from build123d import *

# Parameters (mm, degrees)
F1_DEPTH = 0.5


with BuildPart() as f1:
    # F0 (on Top) → F1 (new body)
    with BuildSketch(Plane.XY):
        with BuildLine():
            ThreePointArc((4.5, 0), (0, -4.5), (-4.5, 0))
            Line((-4.5, 0), (-4.5, 4.834927))
            Line((-4.5, 4.834927), (-11.980261, 4.834927))
            Line((-11.980261, 4.834927), (-14.539381, 0))
            Line((-14.539381, 0), (-14.539381, -15))
            Line((-14.539381, -15), (0, -15))
            Line((0, -15), (14.539381, -15))
            Line((14.539381, -15), (14.539381, 0))
            Line((14.539381, 0), (11.980261, 4.834927))
            Line((11.980261, 4.834927), (4.5, 4.834927))
            Line((4.5, 4.834927), (4.5, 0))
        make_face()
    extrude(amount=F1_DEPTH)


solid = f1.part
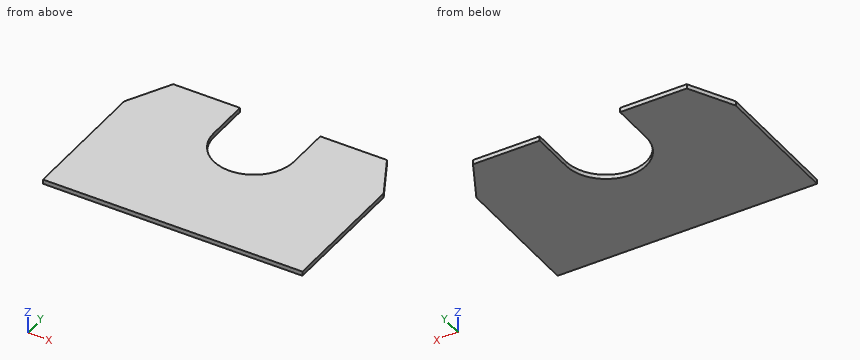
Model file for the job. Use its own axes, mm. Give positions to 0.01 mm unless a question says otherwise; leave off trailing zeros. Order: outer loops, then holes, each group sorted by start corner. A loop starts at its lowest first (then second) coordinate and runs counter-clockwise, first axis right, second up. Notation, with made-up numbers: (-17, 63) - (5, 63) arc R20 cw to (5, 67) - close; hole circle Ø5 at (51, 70.25). An arc over 180 degrees is marked (long way). Write item = value, one per line. Start each with the question number.
1. Cut at D-D, the plane y = -2.5. List the corners of the cut face in (x, z).
2. Probe line 1 along X through (y, z) = (2, 0.25); line 2 along X through (y, z) = (-4, 0.4); line 3 along Y through (x, z) = (-2, 0.15). List the from-to ranges inside material, lowest first.
3. Cut at C-C, the plane x = 0. List the corners of the cut face in (y, z).
4. Cut at A-A, the plane z = 0.35. List the corners of the cut face in (x, y), and give its area (3 significant figures).
5. Cut at B-B, the plane y = 1.25. List the corners of the cut face in (x, z), and give its area (3 significant figures).
Taken from the geometry:
q1.outline = (-14.54, 0) - (-3.74, 0) - (-3.74, 0.5) - (-14.54, 0.5) - close; (3.74, 0) - (14.54, 0) - (14.54, 0.5) - (3.74, 0.5) - close
q2.line_1 = -13.48 to -4.5, 4.5 to 13.48
q2.line_2 = -14.54 to -2.06, 2.06 to 14.54
q2.line_3 = -15 to -4.03
q3.outline = (-15, 0) - (-4.5, 0) - (-4.5, 0.5) - (-15, 0.5) - close
q4.outline = (-14.54, -15) - (14.54, -15) - (14.54, 0) - (11.98, 4.83) - (4.5, 4.83) - (4.5, 0) arc R4.5 cw to (-4.5, 0) - (-4.5, 4.83) - (-11.98, 4.83) - (-14.54, 0) - close
q4.area = 489 mm²
q5.outline = (-13.88, 0) - (-4.5, 0) - (-4.5, 0.5) - (-13.88, 0.5) - close; (4.5, 0) - (13.88, 0) - (13.88, 0.5) - (4.5, 0.5) - close
q5.area = 9.38 mm²
